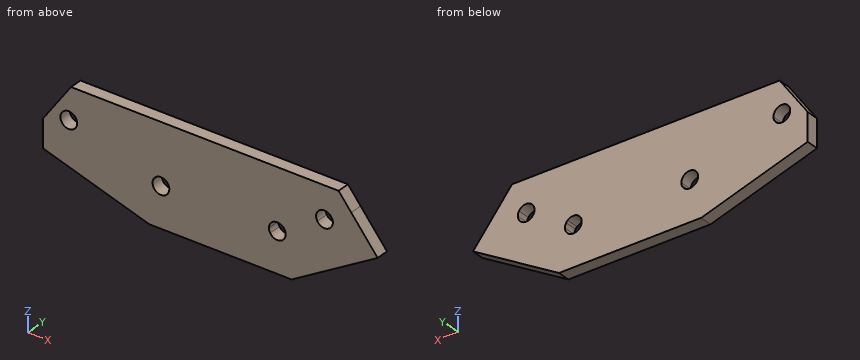
```python
from build123d import *

# Parameters (mm, degrees)
F1_DEPTH = 4.7625


with BuildPart() as f1:
    # F0 (on Front) → F1 (new body)
    with BuildSketch(Plane.XZ):
        with BuildLine():
            Line((26.4038386983, 2.564510672), (44.8625854758, 23.0650258511))
            Line((44.8625854758, 23.0650258511), (-53.9749003947, 23.0650258511))
            Line((-53.9749003947, 23.0650258511), (-64.6206509769, 7.9856580123))
            Line((-64.6206509769, 7.9856580123), (-64.6206509769, -2.6557157676))
            Line((-64.6206509769, -2.6557157676), (-24.221339656, -15.0349741489))
            Line((-24.221339656, -15.0349741489), (-1.1206509769, -15.0349741489))
            Line((-1.1206509769, -15.0349741489), (-1.1206509769, -5.5099741489))
            Line((-1.1206509769, -5.5099741489), (-16.828311902, -0.6967932604))
            ThreePointArc((-16.828311902, -0.6967932604), (-20.8027443302, -2.8306539415), (-22.8994068913, 1.1635269053))
            ThreePointArc((-22.8994068913, 1.1635269053), (-19.3876033028, 3.3427731008), (-16.6975437083, 0.2050258511))
            Line((-16.6975437083, 0.2050258511), (-0.8225437083, 0.2050258511))
            Line((-0.8225437083, 0.2050258511), (21.1043490231, 0.2050258511))
            ThreePointArc((21.1043490231, 0.2050258511), (22.9879601813, 3.1055326791), (26.4038386983, 2.564510672))
        make_face()
        with BuildLine():
            ThreePointArc((-51.6566210989, 10.9482761359), (-51.6916443202, 10.4779881079), (-51.7959413063, 10.018075514))
            ThreePointArc((-51.7959413063, 10.018075514), (-57.9715978776, 11.4185641639), (-51.6566210989, 10.9482761359))
        make_face(mode=Mode.SUBTRACT)
        with BuildLine():
            ThreePointArc((21.556808984, -1.4284981724), (21.219554126, -0.6424882714), (21.1043490231, 0.2050258511))
            Line((21.1043490231, 0.2050258511), (-0.8225437083, 0.2050258511))
            Line((-0.8225437083, 0.2050258511), (-16.6975437083, 0.2050258511))
            ThreePointArc((-16.6975437083, 0.2050258511), (-16.7304058226, -0.2505995516), (-16.828311902, -0.6967932604))
            Line((-16.828311902, -0.6967932604), (-1.1206509769, -5.5099741489))
            Line((-1.1206509769, -5.5099741489), (9.3876935245, -8.7299674481))
            Line((9.3876935245, -8.7299674481), (21.556808984, -1.4284981724))
        make_face()
        with BuildLine():
            Line((52.3552192636, 17.0505479954), (47.5451759994, 23.0650258511))
            Line((47.5451759994, 23.0650258511), (44.8625854758, 23.0650258511))
            Line((44.8625854758, 23.0650258511), (26.4038386983, 2.564510672))
            ThreePointArc((26.4038386983, 2.564510672), (26.7298957035, 2.2237992329), (27.0018890622, 1.8385498746))
            Line((27.0018890622, 1.8385498746), (39.4622261253, 9.3147521124))
            ThreePointArc((39.4622261253, 9.3147521124), (40.551242141, 13.670816175), (44.9073062036, 12.5818001594))
            Line((44.9073062036, 12.5818001594), (52.3552192636, 17.0505479954))
        make_face()
        Polygon((-1.1206509769, -5.5099741489), (-1.1206509769, -15.0349741489), (9.3876935245, -8.7299674481), align=None)
        with BuildLine():
            Line((62.3602304878, 4.5402824637), (52.3552192636, 17.0505479954))
            Line((52.3552192636, 17.0505479954), (44.9073062036, 12.5818001594))
            ThreePointArc((44.9073062036, 12.5818001594), (45.2445610615, 11.7957902584), (45.3597661644, 10.9482761359))
            ThreePointArc((45.3597661644, 10.9482761359), (43.032280287, 7.8884812388), (39.4622261253, 9.3147521124))
            Line((39.4622261253, 9.3147521124), (27.0018890622, 1.8385498746))
            ThreePointArc((27.0018890622, 1.8385498746), (27.3391439202, 1.0525399736), (27.4543490231, 0.2050258511))
            ThreePointArc((27.4543490231, 0.2050258511), (25.1268631456, -2.854769046), (21.556808984, -1.4284981724))
            Line((21.556808984, -1.4284981724), (9.3876935245, -8.7299674481))
            Line((9.3876935245, -8.7299674481), (-1.1206509769, -15.0349741489))
            Line((-1.1206509769, -15.0349741489), (29.7348028, -15.0349741489))
            Line((29.7348028, -15.0349741489), (62.3602304878, 4.5402824637))
        make_face()
    extrude(amount=F1_DEPTH)


solid = f1.part
```
Design review of the part built by this model. Coordinates are the model's own, in mm. Give positions to 0.01 mm unless a question says otherwise; leave off trailing zeros. Order: outer loops, then holes, each group sorted by start corner. A loop starts at its lowest first (then second) coordinate and runs counter-clockwise, first axis right, second up. Notation, with made-up numbers: (75.5, -12.5) -> (86.5, -12.5) arc R4 ccw to (86.5, -6.5) -> close; hole circle Ø2 at (31, -14.5). An arc over 180 degrees is marked (long way). Write item = value, one per line. Start each with the question number.
(1) We need section D-D on z = -9.5. Write out the cut boundary in (x, y).
(2) We need section A-A on y = -1.25. State how many separate pieces and enclosed holes the cut face has, plus the area to 3 significant figures.
(3) We need section B-B on x = -56. Write out the cut boundary in (y, z).
(4) We need section C-C on x = 36. Write out the cut boundary in (y, z).
(5) For pin 1 (4 mm diameter, centred on x = -54.83, z = 10.95, fed in from +Y), flat-tipped, find the tip position at first contact; note if it passes through.
(6) To check wall thickness, follow line 1 along X through (y, z) = (-0.45, 13); line 2 along X through (y, z) = (-0.8, 9.5); line 3 along Z through (x, y) = (21.5, -1.1). State the ranges of each line that lie inside material, in increasing order.
Numbers:
q1.outline = (-42.28, -4.76) -> (38.96, -4.76) -> (38.96, 0) -> (-42.28, 0) -> close
q2.separate_pieces = 1
q2.enclosed_holes = 4
q2.area = 3,920 mm^2
q3.outline = (-4.76, -5.3) -> (0, -5.3) -> (0, 8) -> (-4.76, 8) -> close; (-4.76, 13.9) -> (0, 13.9) -> (0, 20.2) -> (-4.76, 20.2) -> close
q4.outline = (-4.76, -11.28) -> (0, -11.28) -> (0, 23.07) -> (-4.76, 23.07) -> close
q5.pin_1 = through
q6.line_1 = -61.08 to -57.25, -52.41 to 39.76, 44.61 to 55.59
q6.line_2 = -63.55 to -57.66, -52.01 to 39.36, 45.01 to 58.39
q6.line_3 = -15.03 to -1.33, 1.74 to 23.07
